```python
from build123d import *

# Parameters (mm, degrees)
F0_W     = 13
F0_H     = 23.5
F1_DEPTH = 8.5
F2_R     = 1.8
F3_DEPTH = 8
F4_W     = 2
F4_H     = 6
F5_DEPTH = 1.6
F6_R     = 0.2


with BuildPart() as f1:
    # F0 (on Top) → F1 (new body)
    with BuildSketch(Plane.XY):
        with Locations((6.5, 11.75)):
            Rectangle(F0_W, F0_H)
    extrude(amount=F1_DEPTH)

    # F2 (on face) → F3 (join)
    with BuildSketch(Plane.XZ):
        with Locations((2.6, 5.2)):
            Circle(F2_R)
        with Locations((10.4, 5.2)):
            Circle(F2_R)
    extrude(amount=F3_DEPTH)

    # F4 (on face) → F5 (join)
    with BuildSketch(Plane.XZ):
        with Locations((6.5, 8.5)):
            Rectangle(F4_W, F4_H)
    extrude(amount=F5_DEPTH)

    # F6
    f6_edges = [f1.edges().sort_by_distance(p)[0] for p in [
        (6.5, 23.5, 0),
        (13, 11.75, 0),
        (0, 11.75, 0),
        (13, 23.5, 4.25),
        (13, 11.75, 8.5),
        (6.5, 23.5, 8.5),
        (0, 11.75, 8.5),
        (0, 23.5, 4.25),
        (0, 0, 4.25),
        (2.75, 0, 8.5),
        (10.25, 0, 8.5),
        (13, 0, 4.25),
        (6.5, 0, 0),
    ]]
    fillet(f6_edges, radius=F6_R)


solid = f1.part
```
Model file for the job. Use its own axes, mm. A direction names the side the tool comes from. Coordinates: 2 decimals unless noted, no trailing zeros. Order: outer loops, then holes, each group sorted by start corner. A loop starts at its lowest first (then second) coordinate and runs counter-clockwise, first axis right, second up. Notation, with made-up numbers: (-25.75, 69.25) -> (-21.75, 69.25) arc R13 cw to (-21.75, 75.25) -> close; hole circle Ø8 at (39, 43.5). An arc over 180 degrees is marked (long way). Answer as a JSON object with one key per item and string values. Group by question number.
1) Which spindle directions (+Z, -Z, +X, -X, +Y, -Y) get a long thin tool onto all of the face, cutting with end or side? Do faces 5 (the face through (6, -1, 5.5)), 6 (the face through (6, -1.6, 9)), 7 (the face through (1.273, -3.944, 6.417)). Say none if no direction does.
2) Cut at D-D, the plane y = -4.5. Write the cut outline in (x, z).
3) Pull direction X, two halves, no side cores. Call faces 1 (the face through (6, 0, 3)), 2 (the face through (6, 0, 10)), 3 (the face through (13, 12, 4)), 4 (the face through (0, 12, 4)): +X half, -X half, draft (parallel to the pull), parting line (faces both ways), or undercut.
4) Cut at A-A, the plane y = 19. Write the cut outline in (x, z).
5) Cut at C-C, the plane z = 5.2. Write the cut outline in (x, y).
6) Flat gauge pins, fed straight in: pin 1 (1.4 mm diameter, centred on y = -0.5, z = 9.5, fed in from -X); pin 2 (1 mm diameter, centred on x = 6, z = 10, fed in from -Y); pin 3 (3 mm diameter, centred on x = 11.5, y = 11, fed in from +Z); pin 4 (5 mm diameter, centred on x = 9, z = 8, fed in from -Y). Where does each tip first touch, or does it go through?
7) Cut at B-B, the plane x = 4.75. Write the cut outline in (y, z), then the cut area to 3 significant figures.
8) Drill centre lines: L1, parallel to Y at x = 6, z = 4.25; L2, parallel to Z at x = 5.25, y = 1.5; L3, parallel to X at y = -7, z = 4. Where is each one in solid material? Low to high.
Check values:
{
 "1": {"face 5": "-Z, -Y", "face 6": "+Z, -Z, -Y", "face 7": "-Y"},
 "2": {"outline": "circle Ø3.6 at (2.6, 5.2); circle Ø3.6 at (10.4, 5.2)"},
 "3": {"face 1": "undercut", "face 2": "draft", "face 3": "+X half", "face 4": "-X half"},
 "4": {"outline": "(0, 0.2) arc R0.2 ccw to (0.2, 0) -> (12.8, 0) arc R0.2 ccw to (13, 0.2) -> (13, 8.3) arc R0.2 ccw to (12.8, 8.5) -> (0.2, 8.5) arc R0.2 ccw to (0, 8.3) -> close"},
 "5": {"outline": "(0, 0.2) arc R0.2 ccw to (0.2, 0) -> (0.8, 0) -> (0.8, -8) -> (4.4, -8) -> (4.4, 0) -> (8.6, 0) -> (8.6, -8) -> (12.2, -8) -> (12.2, 0) -> (12.8, 0) arc R0.2 ccw to (13, 0.2) -> (13, 23.3) arc R0.2 ccw to (12.8, 23.5) -> (0.2, 23.5) arc R0.2 ccw to (0, 23.3) -> close"},
 "6": {"pin 1": "stops at x = 5.5", "pin 2": "stops at y = -1.6", "pin 3": "stops at z = 8.5", "pin 4": "stops at y = -8"},
 "7": {"outline": "(0, 0.2) arc R0.2 ccw to (0.2, 0) -> (23.3, 0) arc R0.2 ccw to (23.5, 0.2) -> (23.5, 8.3) arc R0.2 ccw to (23.3, 8.5) -> (0.2, 8.5) arc R0.2 ccw to (0, 8.3) -> close", "area": "200 mm²"},
 "8": {"L1": "y = 0 to 23.5", "L2": "z = 0 to 8.5", "L3": "x = 1.26 to 3.94, 9.06 to 11.74"}
}
